from build123d import *

# Parameters (mm, degrees)
SKETCH1_R               = 6
BOSS_EXTRUDE1_DEPTH     = 5
SKETCH1_W               = 66
SKETCH1_H               = 6
BOSS_EXTRUDE1_2_DEPTH   = 5
SKETCH1_4_W             = 2.5
SKETCH1_4_H             = 34
BOSS_EXTRUDE2_DEPTH     = 10
CUT_EXTRUDE1_DEPTH      = 51.418870475
CUT_EXTRUDE1_DEPTH_BACK = 51.418870475
SKETCH2_R               = 3
BOSS_EXTRUDE3_DEPTH     = 46
SKETCH3_W               = 41
SKETCH3_H               = 3
BOSS_EXTRUDE4_DEPTH     = 41
SKETCH4_R               = 3
SKETCH4_R_2             = 1.5
CUT_EXTRUDE2_DEPTH      = 6


with BuildPart() as part:
    # Sketch1 → Boss-Extrude1 (new body)
    with BuildSketch(Plane(origin=(0, 0, 0), x_dir=(0, 0, -1), z_dir=(1, 0, 0))):
        Polygon((-28, 12), (-28, 7), (-30.5, 7), (-30.5, -13), (30.5, -13), (30.5, 7), (28, 7), (28, 12), align=None)
        with Locations((-15.5, 0)):
            Circle(SKETCH1_R, mode=Mode.SUBTRACT)
        with Locations((15.5, 0)):
            Circle(SKETCH1_R, mode=Mode.SUBTRACT)
    extrude(amount=BOSS_EXTRUDE1_DEPTH)

    # Sketch1<4> → Boss-Extrude2 (add)
    with BuildSketch(Plane(origin=(0, 0, 0), x_dir=(0, 0, -1), z_dir=(1, 0, 0))):
        with Locations((0, -5)):
            Rectangle(SKETCH1_4_W, SKETCH1_4_H)
        Polygon((-33, 4), (-33, -22), (-30.5, -22), (-30.5, 7), (-43, 7), (-43, 4), align=None)
        Polygon((30.5, -22), (33, -22), (33, 4), (43, 4), (43, 7), (30.5, 7), align=None)
    extrude(amount=-BOSS_EXTRUDE2_DEPTH)


with BuildPart() as body_2:
    # Sketch1 → Boss-Extrude1 2 (new body)
    with BuildSketch(Plane(origin=(0, 0, 0), x_dir=(0, 0, -1), z_dir=(1, 0, 0))):
        with Locations((0, -19)):
            Rectangle(SKETCH1_W, SKETCH1_H)
    extrude(amount=BOSS_EXTRUDE1_2_DEPTH)



with BuildPart() as boss_extrude2_piece_1:
    # of the separate pieces the step leaves, piece 1, a body of its own (boss_extrude2_pieces)
    add(part.part.solids().sort_by_distance((0, 7, -28))[0])


with BuildPart() as boss_extrude2_piece_2:
    # of the separate pieces the step leaves, piece 2, a body of its own (boss_extrude2_pieces)
    add(part.part.solids().sort_by_distance((0, -22, 30.5))[0])


with BuildPart() as boss_extrude2_piece_3:
    # of the separate pieces the step leaves, piece 3, a body of its own (boss_extrude2_pieces)
    add(part.part.solids().sort_by_distance((-10, 7, -30.5))[0])


with BuildPart() as cut_extrude1_tool:
    # Sketch2 → Cut-Extrude1 (new, two sides: drawn at the far end of the back side and taken through both)
    with BuildSketch(Plane.XY.offset(1.25).offset(-CUT_EXTRUDE1_DEPTH_BACK)):
        with Locations((-5, -15.5)):
            Circle(SKETCH2_R)
    extrude(amount=CUT_EXTRUDE1_DEPTH + CUT_EXTRUDE1_DEPTH_BACK)


with BuildPart() as boss_extrude2_piece_1_1:
    add(boss_extrude2_piece_1.part)

    # Cut-Extrude1: cut by cut_extrude1_tool
    add(cut_extrude1_tool.part, mode=Mode.SUBTRACT)


with BuildPart() as boss_extrude2_piece_2_1:
    add(boss_extrude2_piece_2.part)

    # Cut-Extrude1: cut by cut_extrude1_tool
    add(cut_extrude1_tool.part, mode=Mode.SUBTRACT)


with BuildPart() as boss_extrude2_piece_3_1:
    add(boss_extrude2_piece_3.part)

    # Cut-Extrude1: cut by cut_extrude1_tool
    add(cut_extrude1_tool.part, mode=Mode.SUBTRACT)


with BuildPart() as body_2_1:
    add(body_2.part)

    add(boss_extrude2_piece_1_1.part)  # Boss-Extrude3 merges Boss-Extrude2 piece 1

    add(boss_extrude2_piece_2_1.part)  # Boss-Extrude3 merges Boss-Extrude2 piece 2

    add(boss_extrude2_piece_3_1.part)  # Boss-Extrude3 merges Boss-Extrude2 piece 3
    # Sketch1<6> → Boss-Extrude3 (add)
    with BuildSketch(Plane(origin=(0, 0, 0), x_dir=(0, 0, -1), z_dir=(1, 0, 0))):
        Polygon((-30.5, -13), (-30.5, 7), (-43, 7), (-43, 4), (-33, 4), (-33, -16), (33, -16), (33, 4), (43, 4), (43, 7), (30.5, 7), (30.5, -13), align=None)
    extrude(amount=BOSS_EXTRUDE3_DEPTH)

    # Sketch3 → Boss-Extrude4 (add)
    with BuildSketch(Plane.XZ.offset(16)):
        with Locations((25.5, 28.5)):
            Rectangle(SKETCH3_W, SKETCH3_H)
    extrude(amount=BOSS_EXTRUDE4_DEPTH)

    # Sketch4 → Cut-Extrude2 (cut)
    with BuildSketch(Plane(origin=(0, 0, 27), x_dir=(-1, 0, 0), z_dir=(0, 0, -1))):
        with Locations((-25.5, -36.5)):
            Circle(SKETCH4_R)
        with Locations((-41.42, -20.58)):
            Circle(SKETCH4_R_2)
        with Locations((-9.58, -20.58)):
            Circle(SKETCH4_R_2)
        with Locations((-9.58, -52.42)):
            Circle(SKETCH4_R_2)
        with Locations((-41.42, -52.42)):
            Circle(SKETCH4_R_2)
    extrude(amount=-CUT_EXTRUDE2_DEPTH, mode=Mode.SUBTRACT)


solid = body_2_1.part
The listing builds one solid part. Answer for the finished solid, in the listing's coordinates (mm). A direction names the side the tool comes from. Coordinates: 2 decimals unless noted, no trailing zeros. Order: outer loops, then holes, each group sorted by start corner. A loop starts at its lowest first (then second) coordinate and runs counter-clockwise, first axis right, second up.
Q1. A cutting plane is placed at D-D, the plane x = 41.42. Write down the section's boundary in (y, z).
Q2. A cutting plane is placed at A-A, the plane z = -15.5. Write down the section's boundary in (x, y).
Q3. Consider line 1 (Y direction, x = 41.42, z = 28.15); line 2 (Y direction, x = 1.5, z = -15.5); line 3 (Z direction, x = 24, y = 3). Determine where each line is inside the solid, lowest interval first.
Q4. A cutting plane is placed at C-C, the plane y = -20.58. Write down the section's boundary in (x, z), and give its area (3 significant figures).
Q5. For a pull along Y with two mould halves and no side action, classify faces 5 (the face through (18, 4, -38)), 6 (the face through (18, -6, -33)), 7 (the face through (8.194, -21.155, 28.479)) as pulls with the +Y half, pulls with the -Y half, needs draft (parallel to the pull), parting line crosses it, or undercut.
Q6. A cutting plane is placed at B-B, the plane x = -5. Write down the section's boundary in (y, z), and give its area (3 significant figures).
Q7. Which of the six approach directions +Z, -Z, +X, -X, +Y, -Y give full straight-line access (tool end or side, diameter ignored) to faces 1 (the face through (5, -39, 28)), 2 (the face through (25, -16, 32)), 3 (the face through (18, -6, 33)), 4 (the face through (-5, -7, -30.5))?
Q8. Given P1, Ø0.9, axis at y = -20, z = 31, coming from the +X side; P2, Ø12, axis at x = 19.5, z = 35, coming from the +Y side; P3, Ø5, axis at x = 15.5, y = -36, coming from the +Z side, each flat-ended and moving along its own axis, determine where each tip first touches the part or whether it passes through.
Answers follow:
1. outline: (-57, 27) - (-53.92, 27) - (-53.92, 30) - (-57, 30) - close; (-50.92, 27) - (-22.08, 27) - (-22.08, 30) - (-50.92, 30) - close; (-19.08, 27) - (-16, 27) - (-16, -33) - (4, -33) - (4, -43) - (7, -43) - (7, -30.5) - (-13, -30.5) - (-13, 30.5) - (7, 30.5) - (7, 43) - (4, 43) - (4, 33) - (-16, 33) - (-16, 30) - (-19.08, 30) - close
2. outline: (0, -22) - (5, -22) - (5, -16) - (46, -16) - (46, -13) - (5, -13) - (5, -6) - (0, -6) - close; (0, 6) - (5, 6) - (5, 12) - (0, 12) - close
3. line 1: y = -57 to -53.92, -50.92 to -22.08, -19.08 to -13
3. line 2: y = -22 to -6, 6 to 12
3. line 3: z = -33 to -30.5, 30.5 to 33
4. outline: (-10, -33) - (5, -33) - (5, 27) - (8.08, 27) - (8.08, 30) - (5, 30) - (5, 33) - (-10, 33) - (-10, 30.5) - (0, 30.5) - (0, 1.25) - (-10, 1.25) - (-10, -1.25) - (0, -1.25) - (0, -30.5) - (-10, -30.5) - close; (11.08, 27) - (39.92, 27) - (39.92, 30) - (11.08, 30) - close; (42.92, 27) - (46, 27) - (46, 30) - (42.92, 30) - close
4. area: 510 mm2
5. face 5: pulls with the -Y half
5. face 6: needs draft
5. face 7: undercut
6. outline: (-22, -33) - (-18.5, -33) - (-18.5, -30.5) - (-22, -30.5) - close; (-22, -1.25) - (-18.5, -1.25) - (-18.5, 1.25) - (-22, 1.25) - close; (-22, 30.5) - (-18.5, 30.5) - (-18.5, 33) - (-22, 33) - close; (-12.5, -33) - (4, -33) - (4, -43) - (7, -43) - (7, -30.5) - (-12.5, -30.5) - close; (-12.5, -1.25) - (12, -1.25) - (12, 1.25) - (-12.5, 1.25) - close; (-12.5, 30.5) - (7, 30.5) - (7, 43) - (4, 43) - (4, 33) - (-12.5, 33) - close
6. area: 245 mm2
7. face 1: +Z, -Z, -X, -Y
7. face 2: +Z, +X, -Y
7. face 3: +Z, +X, -X, -Y
7. face 4: -X, +Y, -Y
8. P1: stops at x = 5
8. P2: stops at y = 7
8. P3: stops at z = 30
